from build123d import *

# Parameters (mm, degrees)
CUT_EXTRUDE2_DEPTH = 47.904157598
CIRPATTERN4_COUNT  = 30


with BuildPart() as part:
    # Sketch1 → Revolve1 (revolve)
    with BuildSketch(Plane.XY, mode=Mode.PRIVATE) as revolve1_sk:
        Polygon((-20, 30), (20, 30), (20, 27.05), (16.95, 27.05), (13.9, 24), (-16.95, 24), (-16.95, 27.05), (-20, 27.05), align=None)
    revolve(revolve1_sk.sketch.rotate(Axis((22, 0, 0), (-1, 0, 0)), 90), axis=Axis((22, 0, 0), (-1, 0, 0)))

    # Sketch6 → Cut-Extrude2 (cut, symmetric)
    with BuildSketch(Plane(origin=(0, 0, 0), x_dir=(0, 0, -1), z_dir=(1, 0, 0))):
        Polygon((-30, 1.75), (-29, 1.172649731), (-29, -1.172649731), (-30, -1.75), align=None)
    cut_extrude2 = extrude(amount=CUT_EXTRUDE2_DEPTH, both=True, mode=Mode.SUBTRACT)

    # CirPattern4: Cut-Extrude2 ×30 about axis
    cirpattern4_axis = Axis((0, 0, 0), (1, 0, 0))
    for i in range(1, CIRPATTERN4_COUNT):
        add(cut_extrude2.rotate(cirpattern4_axis, i * 360 / CIRPATTERN4_COUNT), mode=Mode.SUBTRACT)


solid = part.part
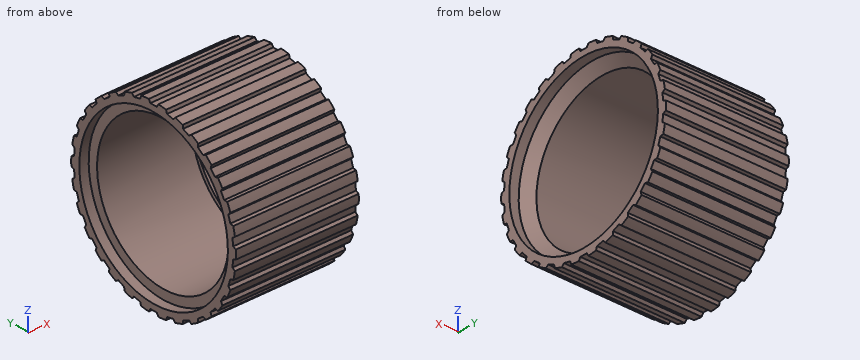
CAD build for the part. Positions are in the model's coordinates, mm. Round coordinates to 2 decimals unless told otherwise and drop trailing zeros. Loops run counter-clockwise (first coordinate to the right, second up) from the corner with the lowest first, then second, coordinate; pieces in that order, holes last.
(1) Cut at B-B (z = 0). Give the cut face in (x, y), plus the area to 3 significant figures.
(2) Cut at A-A (y = 0). Give the cut face in (x, z).
(3) Drop flat-ended pins along their axis: pin 1 (1 mm diameter, centred on x = 5, y = -14, fed in from -Z); pin 2 (1 mm diameter, centred on x = 13.5, y = 11, fed in from +Z); pin 3 (0.9 mm diameter, centred on x = -8, y = -26.5, fed in from +Z). Give the stop position or say it passes through.
(4) Wall check: line 1 along Y through (x, z) = (-1, 0); line 2 along Y through (x, z) = (-19.4, 0); line 3 along Z through (x, y) = (-0.5, 17.5). Give the ranges that are in metal, low to high.
Findings below:
1. outline: (-20, -30) - (20, -30) - (20, -27.05) - (16.95, -27.05) - (13.9, -24) - (-16.95, -24) - (-16.95, -27.05) - (-20, -27.05) - close; (-20, 27.05) - (-16.95, 27.05) - (-16.95, 24) - (13.9, 24) - (16.95, 27.05) - (20, 27.05) - (20, 30) - (-20, 30) - close
1. area: 433 mm2
2. outline: (-20, -29) - (20, -29) - (20, -27.05) - (16.95, -27.05) - (13.9, -24) - (-16.95, -24) - (-16.95, -27.05) - (-20, -27.05) - close; (-20, 27.05) - (-16.95, 27.05) - (-16.95, 24) - (13.9, 24) - (16.95, 27.05) - (20, 27.05) - (20, 29) - (-20, 29) - close
3. pin 1: stops at z = -26.66
3. pin 2: stops at z = 28.1
3. pin 3: stops at z = 13.48
4. line 1: y = -30 to -24, 24 to 30
4. line 2: y = -30 to -27.05, 27.05 to 30
4. line 3: z = -23.13 to -16.42, 16.42 to 23.13
